from build123d import *

# Parameters (mm, degrees)
BOSS_EXTRUDE1_DEPTH = 50
SKETCH3_R           = 11
CUT_EXTRUDE1_DEPTH  = 20
CUT_EXTRUDE2_DEPTH  = 4
BOSS_EXTRUDE2_DEPTH = 4
SKETCH7_R           = 1.5
CUT_EXTRUDE3_DEPTH  = 4


with BuildPart() as part:
    # Sketch1 → Boss-Extrude1 (new body)
    with BuildSketch(Plane(origin=(0, 0, 0), x_dir=(0, 0, -1), z_dir=(1, 0, 0))):
        Polygon((0, 0), (0, 50), (3, 50), (3, 3), (50, 3), (50, 0), align=None)
    extrude(amount=BOSS_EXTRUDE1_DEPTH)

    # Sketch3 → Cut-Extrude1 (cut)
    with BuildSketch(Plane(origin=(0, 0, -3), x_dir=(-1, 0, 0), z_dir=(0, 0, -1))):
        with Locations((-25, 26.5)):
            Circle(SKETCH3_R)
    extrude(amount=-CUT_EXTRUDE1_DEPTH, mode=Mode.SUBTRACT)

    # Sketch4 → Cut-Extrude2 (cut, through all)
    with BuildSketch(Plane(origin=(0, 3, 0), x_dir=(1, 0, 0), z_dir=(0, 1, 0))):
        with BuildLine():
            Line((7.5, 14), (7.5, 39))
            ThreePointArc((7.5, 39), (10, 41.5), (12.5, 39))
            Line((12.5, 39), (12.5, 14))
            ThreePointArc((12.5, 14), (10, 11.5), (7.5, 14))
        make_face()
        with BuildLine():
            Line((42.5, 14), (42.5, 39))
            ThreePointArc((42.5, 39), (40, 41.5), (37.5, 39))
            Line((37.5, 39), (37.5, 14))
            ThreePointArc((37.5, 14), (40, 11.5), (42.5, 14))
        make_face()
    extrude(amount=-CUT_EXTRUDE2_DEPTH, mode=Mode.SUBTRACT)

    # Sketch6 → Boss-Extrude2 (add)
    with BuildSketch(Plane(origin=(50, 0, 0), x_dir=(0, 0, -1), z_dir=(1, 0, 0))):
        Polygon((3, 3), (18, 3), (3, 18), align=None)
    boss_extrude2 = extrude(amount=-BOSS_EXTRUDE2_DEPTH)

    # Mirror1: Boss-Extrude2 across plane
    add(boss_extrude2.mirror(Plane(origin=(25, 0, 0), x_dir=(0, 0, 1), z_dir=(1, 0, 0))))

    # Sketch7 → Cut-Extrude3 (cut, through all)
    with BuildSketch(Plane(origin=(0, 0, -3), x_dir=(-1, 0, 0), z_dir=(0, 0, -1))):
        with Locations((-40.556349186, 42.056349186)):
            Circle(SKETCH7_R)
        with Locations((-9.443650814, 42.056349186)):
            Circle(SKETCH7_R)
        with Locations((-40.556349186, 10.943650814)):
            Circle(SKETCH7_R)
        with Locations((-9.443650814, 10.943650814)):
            Circle(SKETCH7_R)
    extrude(amount=-CUT_EXTRUDE3_DEPTH, mode=Mode.SUBTRACT)


solid = part.part
Could you check a few things on this model? Use its own coordinates, in mm. A direction names the side the tool comes from. Coordinates: 2 decimals unless noted, no trailing zeros. Order: outer loops, then holes, each group sorted by start corner. A loop starts at its lowest first (then second) coordinate and runs counter-clockwise, first axis right, second up.
Q1. Which directions (+Z, -Z, +X, -X, +Y, -Y) give clear straight access to the entire face, cutting with the end or side of a thin tool? Please do faces 4 (the cylindrical face through (8.637, 43.321, -1.521)), 5 (the flat face through (12.5, 2, -27)).
Q2. Thinking about a two-plate mould opening in Z: for faces 1 (the flat face through (46, 7, -7)), 2 (the flat face through (37.5, 2, -27)), 3 (the flat face through (48, 10, -11)), which applies, released by +Z, released by -Z, zero draft, split by the parting line, or undercut?
Q3. Suppose I cut it at B-B on z = -22. Please give me the cut outline in (x, y), and give its area (3 significant figures).
Q4. Suppose I cut it at D-D on x = 41. Please give me the cut outline in (y, z).
Q5. Will these pins go through, and if not, where does the flat tip stop? pin 1 (5 mm diameter, centred on x = 36.5, y = 28.5, fed in from -Z); pin 2 (23.5 mm diameter, centred on x = 23, z = -24.5, fed in from +Y).
Q6. Suppose I cut it at A-A on x = 25. Please give me the cut outline in (y, z), and give its area (3 significant figures).
Q7. Suppose I cut it at C-C on y = 26.5. Please give me the cut outline in (x, z).
Q8. Please list where these lines run through material, in increasing order: L1, parallel to Y at x = 25, z = -1.6; L2, parallel to Y at x = 34, z = -5; L3, parallel to Z at x = 9.5, y = 25.
Answer:
1. face 4: +Z, -Z
1. face 5: +Y, -Y
2. face 1: zero draft
2. face 2: undercut
2. face 3: released by -Z
3. outline: (0, 0) - (7.5, 0) - (7.5, 3) - (0, 3) - close; (12.5, 0) - (37.5, 0) - (37.5, 3) - (12.5, 3) - close; (42.5, 0) - (50, 0) - (50, 3) - (42.5, 3) - close
3. area: 120 mm2
4. outline: (0, -50) - (3, -50) - (3, -41.29) - (0, -41.29) - close; (0, -11.71) - (3, -11.71) - (3, -3) - (9.51, -3) - (9.51, 0) - (0, 0) - close; (12.38, -3) - (40.62, -3) - (40.62, 0) - (12.38, 0) - close; (43.49, -3) - (50, -3) - (50, 0) - (43.49, 0) - close
5. pin 1: stops at z = -3
5. pin 2: stops at y = 3
6. outline: (0, -50) - (3, -50) - (3, -3) - (15.5, -3) - (15.5, 0) - (0, 0) - close; (37.5, -3) - (50, -3) - (50, 0) - (37.5, 0) - close
6. area: 225 mm2
7. outline: (0, -3) - (14, -3) - (14, 0) - (0, 0) - close; (36, -3) - (50, -3) - (50, 0) - (36, 0) - close
8. L1: y = 0 to 15.5, 37.5 to 50
8. L2: y = 0 to 3
8. L3: z = -3 to 0
